Part model, mm, in its own coordinate system. A direction names the side the tool comes from. Give positions to 0.01 mm unless a question says otherwise; leave off trailing zeros. Write each loop counter-clockwise with the first axis right and the second up, starting at its lowest first coordinate (ties: lowest second). Pieces come first, ordered by that corner, then holes. Notation, with made-up numbers: (80, -32.75) - (94, -32.75) arc R21 cw to (94, -14.75) - close; hole circle Ø7 at (89, 23). An arc over 180 degrees is marked (long way). Answer in a Markdown table with one row per item. Add a question column.
1. Pull direction Y, two halves, no side cores. Call faces 1 (the flat face through (79.932, 156.542, 26.084)), 2 (the cylindrical face through (71.826, 55.468, 25.916)), 3 (the flat face through (23.26, -61, 26)), 4 (the flat face through (97.844, 187.232, 26.084)): released by +Y, released by -Y, zero draft, split by the parting line, or undercut.
2. Band-saw the part on B-B on y = 111. Write the cut outline in (x, z), plus the area to 3 significant figures.
3. Probe line 1 along X through (y, z) = (-14, 31); line 2 along Y through (x, z) = (29.5, 24.25); line 3 along X through (y, z) = (129, 28.75). List the from-to ranges inside material, lowest first.
4. Drop flat-ended pins along their axis: pin 1 Ø4 at (x, z) = (108.5, 28) entering from +Y; pin 2 Ø3 at (y, z) = (191, 28) entering from -X; pin 3 Ø3 at (y, z) = (-46.5, 29.5) entering from +X. Give the stop position or say it passes through.
5. Band-saw the part on A-A on z = 22. Write the cut outline in (x, y).
6. Band-saw the part on C-C on x = 113. Write the cut outline in (y, z).
7. Which spindle directions (+Z, -Z, +X, -X, +Y, -Y) get a long thin tool onto all of the face, cutting with end or side? Do faces 5 (the flat face through (29, -43.001, 26)), 6 (the flat face through (73, 77, 32)), 7 (the flat face through (37.89, 77.48, 25.92)). Say none if no direction does.
Autodesk Inventor part; units mm, degrees
ref_plane "YZ Plane" through (0, 0, 0) normal (1, 0, 0) x (0, 1, 0)
ref_plane "XZ Plane" through (0, 0, 0) normal (0, 1, 0) x (-1, 0, 0)
ref_plane "XY Plane" through (0, 0, 0) normal (0, 0, 1) x (1, 0, 0)
ref_plane "Work Plane1" through (0, 0, 20) normal (0, 0, 1) x (1, 0, 0)
sketch "Sketch1" plane through (0, 0, 20) normal (0, 0, 1) x (1, 0, 0)
  circle A0 centre (68.2595, 214.6541) radius 4
  line L0 (64.2595, -185.3459) -> (64.2595, -225.3459)
  arc A1 (72.2595, -185.3459) -> (64.2595, -185.3459) centre (68.2595, -185.3459) ccw
  line L1 (72.2595, -225.3459) -> (72.2595, -185.3459)
  arc A2 (64.2595, -225.3459) -> (72.2595, -225.3459) centre (68.2595, -225.3459) ccw
  line L2 (-101.2595, 230.5421) -> (-90.8671, 224.5421)
  line L3 (-90.8671, 224.5421) -> (-108.8671, 193.3652)
  line L4 (-108.8671, 193.3652) -> (-119.2595, 199.3652)
  line L5 (-137.2595, 168.1883) -> (-119.2595, 199.3652)
  line L6 (-137.2595, 168.1883) -> (-106.0825, 150.1883)
  line L7 (-106.0825, 150.1883) -> (-112.0825, 139.796)
  line L8 (-80.9056, 121.796) -> (-112.0825, 139.796)
  line L9 (-80.9056, 121.796) -> (-74.9056, 132.1883)
  line L10 (-74.9056, 132.1883) -> (-43.7287, 114.1883)
  line L11 (-43.7287, 114.1883) -> (-49.7287, 103.796)
  line L12 (-18.5518, 85.796) -> (-49.7287, 103.796)
  line L13 (-18.5518, 85.796) -> (-12.5518, 96.1883)
  line L14 (-12.5518, 96.1883) -> (18.6251, 78.1883)
  line L15 (18.6251, 78.1883) -> (12.6251, 67.796)
  line L16 (23.2595, 61.6562) -> (12.6251, 67.796)
  line L17 (23.2595, -7.001) -> (23.2595, 61.6562)
  line L18 (23.2595, -7.001) -> (35.2595, -7.001)
  line L19 (35.2595, -7.001) -> (35.2595, -43.001)
  line L20 (35.2595, -43.001) -> (23.2595, -43.001)
  line L21 (23.2595, -79.001) -> (23.2595, -43.001)
  line L22 (23.2595, -79.001) -> (35.2595, -79.001)
  line L23 (35.2595, -79.001) -> (35.2595, -115.001)
  line L24 (35.2595, -115.001) -> (23.2595, -115.001)
  line L25 (23.2595, -151.001) -> (23.2595, -115.001)
  line L26 (23.2595, -151.001) -> (35.2595, -151.001)
  line L27 (35.2595, -151.001) -> (35.2595, -187.001)
  line L28 (35.2595, -187.001) -> (23.2595, -187.001)
  line L29 (23.2595, -223.001) -> (23.2595, -187.001)
  line L30 (23.2595, -223.001) -> (35.2595, -223.001)
  line L31 (35.2595, -223.001) -> (35.2595, -259.001)
  line L32 (35.2595, -259.001) -> (23.2595, -259.001)
  line L33 (23.2595, -295.001) -> (23.2595, -259.001)
  line L34 (23.2595, -295.001) -> (35.2595, -295.001)
  line L35 (35.2595, -295.001) -> (35.2595, -331.001)
  line L36 (105.7595, -290.2979) -> (35.2595, -331.001)
  arc A3 (105.7595, -290.2979) -> (143.2595, -225.3459) centre (68.2595, -225.3459) ccw
  line L37 (143.2595, -185.3459) -> (143.2595, -225.3459)
  arc A4 (143.2595, -185.3459) -> (125.3012, -136.6505) centre (68.2595, -185.3459) ccw
  arc A5 (114.6586, -107.7924) -> (125.3012, -136.6505) centre (159.1055, -107.7924) ccw
  line L38 (114.6586, 129.2663) -> (114.6586, -107.7924)
  arc A6 (5.9066, 302.615) -> (62.9654, 289.467) centre (55.9066, 389.2175) ccw
  line L39 (-43.2595, 331.001) -> (5.9066, 302.615)
  line L40 (-65.2595, 292.8959) -> (-43.2595, 331.001)
  line L41 (-65.2595, 292.8959) -> (-54.8671, 286.8959)
  line L42 (-54.8671, 286.8959) -> (-72.8671, 255.719)
  line L43 (-72.8671, 255.719) -> (-83.2595, 261.719)
  line L44 (-101.2595, 230.5421) -> (-83.2595, 261.719)
  circle A7 centre (28.2595, 174.6541) radius 30
  line L45 (71.9456, 130.5421) -> (61.5533, 136.5421)
  line L46 (61.5533, 136.5421) -> (79.5533, 167.719)
  line L47 (79.5533, 167.719) -> (89.9456, 161.719)
  line L48 (89.9456, 161.719) -> (71.9456, 130.5421)
  line L49 (40.4552, 75.9992) -> (71.9456, 130.5421)
  line L50 (40.4552, 75.9992) -> (30.0629, 81.9992)
  line L51 (30.0629, 81.9992) -> (61.5533, 136.5421)
  line L52 (61.5533, 136.5421) -> (71.9456, 130.5421)
  line L53 (40.4552, 75.9992) -> (71.9456, 130.5421)
  line L54 (35.2595, 78.999) -> (35.2595, -6.251)
  line L55 (35.2595, -6.251) -> (23.2595, -6.251)
  line L56 (23.2595, 78.999) -> (23.2595, -6.251)
  line L57 (35.2595, 78.999) -> (23.2595, 78.999)
  line L58 (89.9456, 161.719) -> (137.3521, 243.8295)
  line L59 (131.6514, 174.8386) -> (110.2726, 142.3196)
  arc A8 (110.2726, 142.3196) -> (63.3739, -36.5254) centre (352.1075, -16.6687) ccw
  arc A9 (35.2595, -79.001) -> (63.3739, -36.5254) centre (21.5733, -39.4001) ccw
  line L60 (119.5533, 237.001) -> (129.9456, 231.001)
  arc A10 (131.6514, 174.8386) -> (129.9456, 231.001) centre (90.7859, 201.7046) ccw
  circle A11 centre (68.2595, 214.6541) radius 4
  line L61 (64.2595, -185.3459) -> (64.2595, -225.3459)
  arc A12 (72.2595, -185.3459) -> (64.2595, -185.3459) centre (68.2595, -185.3459) ccw
  line L62 (72.2595, -225.3459) -> (72.2595, -185.3459)
  arc A13 (64.2595, -225.3459) -> (72.2595, -225.3459) centre (68.2595, -225.3459) ccw
  line L63 (-101.2595, 230.5421) -> (-90.8671, 224.5421)
  line L64 (-90.8671, 224.5421) -> (-108.8671, 193.3652)
  line L65 (-108.8671, 193.3652) -> (-119.2595, 199.3652)
  line L66 (-137.2595, 168.1883) -> (-119.2595, 199.3652)
  line L67 (-137.2595, 168.1883) -> (-106.0825, 150.1883)
  line L68 (-106.0825, 150.1883) -> (-112.0825, 139.796)
  line L69 (-80.9056, 121.796) -> (-112.0825, 139.796)
  line L70 (-80.9056, 121.796) -> (-74.9056, 132.1883)
  line L71 (-74.9056, 132.1883) -> (-43.7287, 114.1883)
  line L72 (-43.7287, 114.1883) -> (-49.7287, 103.796)
  line L73 (-18.5518, 85.796) -> (-49.7287, 103.796)
  line L74 (-18.5518, 85.796) -> (-12.5518, 96.1883)
  line L75 (-12.5518, 96.1883) -> (18.6251, 78.1883)
  line L76 (18.6251, 78.1883) -> (12.6251, 67.796)
  line L77 (23.2595, 61.6562) -> (12.6251, 67.796)
  line L78 (23.2595, -7.001) -> (23.2595, 61.6562)
  line L79 (23.2595, -7.001) -> (35.2595, -7.001)
  line L80 (35.2595, -7.001) -> (35.2595, -43.001)
  line L81 (35.2595, -43.001) -> (23.2595, -43.001)
  line L82 (23.2595, -79.001) -> (23.2595, -43.001)
  line L83 (23.2595, -79.001) -> (35.2595, -79.001)
  line L84 (35.2595, -79.001) -> (35.2595, -115.001)
  line L85 (35.2595, -115.001) -> (23.2595, -115.001)
  line L86 (23.2595, -151.001) -> (23.2595, -115.001)
  line L87 (23.2595, -151.001) -> (35.2595, -151.001)
  line L88 (35.2595, -151.001) -> (35.2595, -187.001)
  line L89 (35.2595, -187.001) -> (23.2595, -187.001)
  line L90 (23.2595, -223.001) -> (23.2595, -187.001)
  line L91 (23.2595, -223.001) -> (35.2595, -223.001)
  line L92 (35.2595, -223.001) -> (35.2595, -259.001)
  line L93 (35.2595, -259.001) -> (23.2595, -259.001)
  line L94 (23.2595, -295.001) -> (23.2595, -259.001)
  line L95 (23.2595, -295.001) -> (35.2595, -295.001)
  line L96 (35.2595, -295.001) -> (35.2595, -331.001)
  line L97 (105.7595, -290.2979) -> (35.2595, -331.001)
  arc A14 (105.7595, -290.2979) -> (143.2595, -225.3459) centre (68.2595, -225.3459) ccw
  line L98 (143.2595, -185.3459) -> (143.2595, -225.3459)
  arc A15 (143.2595, -185.3459) -> (125.3012, -136.6505) centre (68.2595, -185.3459) ccw
  arc A16 (114.6586, -107.7924) -> (125.3012, -136.6505) centre (159.1055, -107.7924) ccw
  line L99 (114.6586, 129.2663) -> (114.6586, -107.7924)
  arc A17 (128.1281, 169.4795) -> (114.6586, 129.2663) centre (181.4216, 129.2663) ccw
  arc A18 (128.1281, 169.4795) -> (62.9654, 289.467) centre (68.2595, 214.6541) ccw
  arc A19 (5.9066, 302.615) -> (62.9654, 289.467) centre (55.9066, 389.2175) ccw
  line L100 (-43.2595, 331.001) -> (5.9066, 302.615)
  line L101 (-65.2595, 292.8959) -> (-43.2595, 331.001)
  line L102 (-65.2595, 292.8959) -> (-54.8671, 286.8959)
  line L103 (-54.8671, 286.8959) -> (-72.8671, 255.719)
  line L104 (-72.8671, 255.719) -> (-83.2595, 261.719)
  line L105 (-101.2595, 230.5421) -> (-83.2595, 261.719)
  circle A20 centre (28.2595, 174.6541) radius 30
  line L106 (71.9456, 130.5421) -> (61.5533, 136.5421)
  line L107 (61.5533, 136.5421) -> (79.5533, 167.719)
  line L108 (79.5533, 167.719) -> (89.9456, 161.719)
  line L109 (89.9456, 161.719) -> (71.9456, 130.5421)
  line L110 (35.2595, -7.001) -> (35.2595, 3.1632)
  line L111 (35.2595, -6.251) -> (35.2595, -79.001)
  point P0 (0, 0)
extrude "Extrusion1" add sketch "Sketch1" along normal blind 12 contours A10 L59 A17 A8 A9 L111 L19 L110 L54 L50 L49 L48 L58 | L59 A17
sketch "Sketch3" plane through (0, 0, 32) normal (0, 0, 1) x (1, 0, 0)
  line L0 (35.2595, 78.999) -> (35.2595, -79.001)
  arc A0 (35.2595, -79.001) -> (63.3739, -36.5254) centre (21.5733, -39.4001) ccw
  arc A1 (110.2726, 142.3196) -> (63.3739, -36.5254) centre (352.1075, -16.6687) ccw
  line L1 (110.2726, 142.3196) -> (131.6514, 174.8386)
  arc A2 (131.6514, 174.8386) -> (129.9456, 231.001) centre (90.7859, 201.7046) ccw
  line L2 (129.9456, 231.001) -> (40.4552, 75.9992)
  line L3 (40.4552, 75.9992) -> (35.2595, 78.999)
  line L4 (35.2595, -79.001) -> (23.2595, -79.001)
  line L5 (23.2595, -79.001) -> (23.2595, -43.001)
  line L6 (23.2595, -43.001) -> (35.2595, -43.001)
  line L7 (35.2595, -43.001) -> (35.2595, -79.001)
  line L8 (129.9456, 231.001) -> (40.4552, 75.9992)
  line L9 (85.2004, 153.5001) -> (102.9679, 184.2742)
  line L10 (102.9679, 184.2742) -> (92.5755, 190.2742)
  line L11 (92.5755, 190.2742) -> (74.8081, 159.5001)
  line L12 (74.8081, 159.5001) -> (85.2004, 153.5001)
  point P0 (0, 0)
  dimension "d2" = 12
  dimension "d3" = 36
  dimension "d4" = 12
extrude "Extrusion2" add sketch "Sketch3" against normal up to surface (12 mm away) contours L0 L4 L5 L6 | L12 L11 L10 L2
sketch "Sketch4" plane through (0, 0, 32) normal (0, 0, 1) x (1, 0, 0)
  line L0 (35.2595, 78.999) -> (35.2595, -43.001)
  line L1 (35.2595, -43.001) -> (23.2595, -43.001)
  line L2 (23.2595, -43.001) -> (23.2595, -79.001)
  line L3 (23.2595, -79.001) -> (35.2595, -79.001)
  arc A0 (35.2595, -79.001) -> (63.3739, -36.5254) centre (21.5733, -39.4001) ccw
  arc A1 (110.2726, 142.3196) -> (63.3739, -36.5254) centre (352.1075, -16.6687) ccw
  line L4 (110.2726, 142.3196) -> (131.6514, 174.8386)
  arc A2 (131.6514, 174.8386) -> (129.9456, 231.001) centre (90.7859, 201.7046) ccw
  line L5 (129.9456, 231.001) -> (102.9679, 184.2742)
  line L6 (102.9679, 184.2742) -> (92.5755, 190.2742)
  line L7 (92.5755, 190.2742) -> (74.8081, 159.5001)
  line L8 (74.8081, 159.5001) -> (85.2004, 153.5001)
  line L9 (85.2004, 153.5001) -> (40.4552, 75.9992)
  line L10 (40.4552, 75.9992) -> (35.2595, 78.999)
  point P0 (0, 0)
properties part number "wooden_stiffener"
Values:
| question | item | result |
|---|---|---|
| 1 | face 1 | undercut |
| 1 | face 2 | undercut |
| 1 | face 3 | zero draft |
| 1 | face 4 | released by +Y |
| 2 | outline | (60.66, 20) - (92.37, 20) - (92.37, 32) - (60.66, 32) - close |
| 2 | area | 381 mm² |
| 3 | line 1 | x = 35.26 to 62.7 |
| 3 | line 2 | y = -79 to -43 |
| 3 | line 3 | x = 71.06 to 102.02 |
| 4 | pin 1 | stops at y = 197.32 |
| 4 | pin 2 | stops at x = 92.13 |
| 4 | pin 3 | stops at x = 63.1 |
| 5 | outline | (23.26, -79) - (35.26, -79) arc R41.9 ccw to (63.37, -36.53) arc R289.42 cw to (110.27, 142.32) - (131.65, 174.84) arc R48.91 ccw to (129.95, 231) - (102.97, 184.27) - (92.58, 190.27) - (74.81, 159.5) - (85.2, 153.5) - (71.95, 130.54) - (40.46, 76) - (35.26, 79) - (35.26, -43) - (23.26, -43) - close |
| 6 | outline | (146.47, 20) - (201.65, 20) - (201.65, 32) - (146.47, 32) - close |
| 7 | face 5 | +Z, -Z, -X, +Y |
| 7 | face 6 | +Z, +X, -X, +Y, -Y |
| 7 | face 7 | +Z, -Z, +Y |
